from build123d import *

# Parameters (mm, degrees)
SKETCH1_W           = 11.25
SKETCH1_H           = 6.1
BOSS_EXTRUDE1_DEPTH = 2
SKETCH2_W           = 10.615
SKETCH2_H           = 2.73
CUT_EXTRUDE1_DEPTH  = 3.81
SKETCH4_R           = 0.309051048
BOSS_EXTRUDE2_DEPTH = 3.81
FILLET1_R           = 0.254


with BuildPart() as part:
    # Sketch1 → Boss-Extrude1 (new body)
    with BuildSketch(Plane(origin=(0, 0, 0), x_dir=(1, 0, 0), z_dir=(0, 1, 0))):
        Rectangle(SKETCH1_W, SKETCH1_H)
    extrude(amount=BOSS_EXTRUDE1_DEPTH)

    # Sketch2 → Cut-Extrude1 (cut)
    with BuildSketch(Plane(origin=(0, 0, -3.05), x_dir=(-1, 0, 0), z_dir=(0, 0, -1))):
        Rectangle(SKETCH2_W, SKETCH2_H)
    extrude(amount=-CUT_EXTRUDE1_DEPTH, mode=Mode.SUBTRACT)

    # Sketch4 → Boss-Extrude2 (add)
    with BuildSketch(Plane(origin=(0, 0, 0.76), x_dir=(-1, 0, 0), z_dir=(0, 0, -1))):
        with Locations(Location((-3.53822, 0.6825, 0), (0, 0, 180))):
            Circle(SKETCH4_R)
        with Locations(Location((-1.76911, 0.6825, 0), (0, 0, 180))):
            Circle(SKETCH4_R)
        with Locations(Location((0, 0.6825, 0), (0, 0, 180))):
            Circle(SKETCH4_R)
        with Locations(Location((1.76911, 0.6825, 0), (0, 0, 180))):
            Circle(SKETCH4_R)
        with Locations(Location((3.53822, 0.6825, 0), (0, 0, 180))):
            Circle(SKETCH4_R)
    extrude(amount=BOSS_EXTRUDE2_DEPTH)

    # Fillet1
    fillet1_edges = [part.edges().sort_by_distance(p)[0] for p in [
        (3.229168952, 0.6825, -3.05),
        (1.460058952, 0.6825, -3.05),
        (-0.309051048, 0.6825, -3.05),
        (-2.078161048, 0.6825, -3.05),
        (-3.847271048, 0.6825, -3.05),
    ]]
    fillet(fillet1_edges, radius=FILLET1_R)


solid = part.part
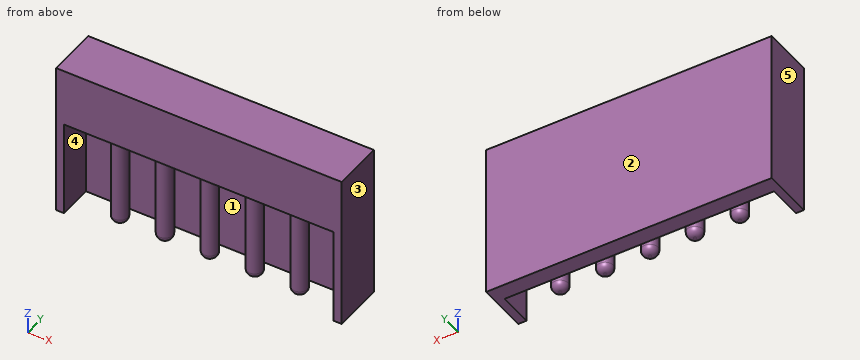
Can you work these out from the model? Positions are in its coordinate system, mm. Face numbers are marked on the shaded views. A direction names the side the tool comes from. Coordinates: 2 decimals unless noted, no trailing zeros. Loops run counter-clockwise (first coordinate to the right, second up) from the corner with the lowest first, then second, coordinate; pieces in that order, holes last. Notation, with made-up numbers: (49.5, 54.5) - (83.5, 54.5) arc R20 ccw to (83.5, 88.5) - close; hole circle Ø10 at (56, 66). An arc over 180 degrees is marked (long way). Answer as a JSON object with one key per item and string values. Group by question number.
Item 1: For pin 1 (1.9 mm diameter, centred on x = -2.5, z = -1, fed in from -Y), with a flat end and sliding along its axis, tell me the tip position at first contact or that it passes through.
Item 2: If we section it at B-B (z = -1.75): State how many separate pieces and enclosed holes the cut face has, plus the area to 3 significant figures.
Item 3: If I drill on L1, parallel to X at y = 0.15, z = -0.5 (1 decimal); L2, parallel to Z at x = 4.25, y = 1.15; L3, parallel to Y at x = 2, z = -1.5 (3 decimals), over which ranges is the centre line in solid material (lowest first)? Write a range as from..to.
Item 4: If we section it at A-A (x = -2.75): List the corners of the cut face in (y, z) for me (3 decimals).
Item 5: On a 3-axis mill with a long thin cutter (end or side, diameter ignored), from which of +Z, -Z, +X, -X, +Y, -Y can I reach the whole of each face in a straight line? I mean the marked faces 4 and 5. Say none if no direction works.
Item 6: If we mould it in two halves opening along Y, with no side actions, what happens to the marked faces 1, 2 and 3? For each: released by +Y, released by -Y, zero draft, split by the parting line, or undercut.
Returned:
{
 "1": {"pin 1": "stops at y = 0.37"},
 "2": {"separate pieces": "6", "enclosed holes": "0", "area": "9.51 mm²"},
 "3": {"L1": "x = -5.6..-5.3, 5.3..5.6", "L2": "z = 0.76..3.05", "L3": "y = 0.477..0.888, 1.365..2"},
 "4": {"outline": "(0, 0.76) - (1.365, 0.76) - (1.365, -3.05) - (2, -3.05) - (2, 3.05) - (0, 3.05) - close"},
 "5": {"face 4": "-Z, -Y", "face 5": "+Z, -Z, -X, +Y, -Y"},
 "6": {"face 1": "undercut", "face 2": "released by +Y", "face 3": "zero draft"}
}
